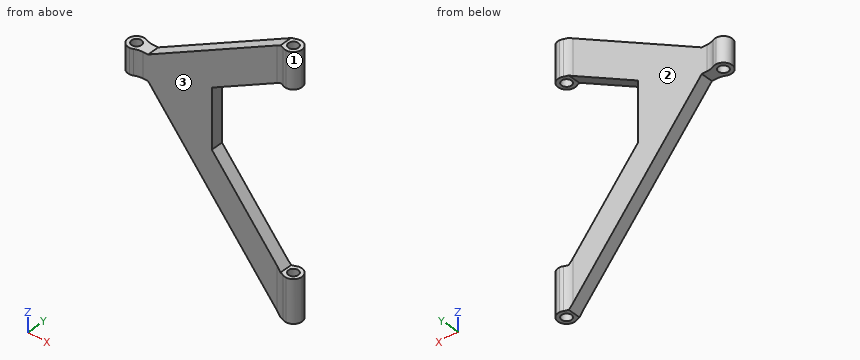
from build123d import *

# Parameters (mm, degrees)
BOSS_EXTRUDE1_DEPTH      = 2.38125
BOSS_EXTRUDE1_DEPTH_BACK = 2.38125
CUT_EXTRUDE1_DEPTH       = 68.891743782
CUT_EXTRUDE1_DEPTH_BACK  = 68.891743782
SKETCH2_R                = 1.375
FILLET2_R                = 2.38125
CUT_EXTRUDE2_DEPTH       = 61.804572212
CUT_EXTRUDE2_DEPTH_BACK  = 61.804572212


with BuildPart() as part:
    # Sketch1 → Boss-Extrude1 (new, two sides: drawn at the far end of the back side and taken through both)
    with BuildSketch(Plane(origin=(0, 0, 0), x_dir=(1, 0, 0), z_dir=(0, 1, 0)).offset(-BOSS_EXTRUDE1_DEPTH_BACK)):
        Polygon((0, 41.898993428), (-37, -2.75), (-44, -2.75), (-44, -9.75), (-37, -9.75), (0, -29.761006572), (4.489108528, -29.761006572), (4.489108528, -19.854089936), (0, -19.854089936), (-19.216520838, -9.461064942), (-19.216520838, 6.902295225), (0, 30.091438809), (4.489108528, 30.091438809), (4.489108528, 41.898993428), align=None)
    extrude(amount=BOSS_EXTRUDE1_DEPTH + BOSS_EXTRUDE1_DEPTH_BACK)

    # Sketch2 → Cut-Extrude1 (cut, two sides: drawn at the far end of the back side and taken through both)
    with BuildSketch(Plane.XY.offset(9.75).offset(-CUT_EXTRUDE1_DEPTH_BACK)):
        with Locations((-41.61875, 0)):
            Circle(SKETCH2_R)
        with Locations((2.107858528, 0)):
            Circle(SKETCH2_R)
    extrude(amount=CUT_EXTRUDE1_DEPTH + CUT_EXTRUDE1_DEPTH_BACK, mode=Mode.SUBTRACT)

    # Fillet2
    fillet2_edges = [part.edges().sort_by_distance(p)[0] for p in [
        (4.489108528, 2.38125, -35.995216119),
        (4.489108528, -2.38125, -35.995216119),
        (4.489108528, -2.38125, 24.807548254),
        (4.489108528, 2.38125, 24.807548254),
        (-44, -2.38125, 6.25),
        (-44, 2.38125, 6.25),
    ]]
    fillet(fillet2_edges, radius=FILLET2_R - 0.0001)  # a hair under: the kernel refuses the full size

    # Sketch3 → Cut-Extrude2 (cut, two sides: drawn at the far end of the back side and taken through both)
    with BuildSketch(Plane.XY.offset(-CUT_EXTRUDE2_DEPTH_BACK)):
        with BuildLine():
            Line((-38.450893086, -1.673565387), (-1.059998386, -1.673565387))
            ThreePointArc((-1.059998386, -1.673565387), (0.043808846, -1.795357088), (1.094509688, -2.154872546))
            ThreePointArc((1.094509688, -2.154872546), (1.588695109, -2.323966632), (2.107858528, -2.38125))
            Line((2.107858528, -2.38125), (2.107858528, -4.833118282))
            Line((2.107858528, -4.833118282), (-41.61875, -4.833118282))
            Line((-41.61875, -4.833118282), (-41.61875, -2.38125))
            ThreePointArc((-41.61875, -2.38125), (-41.099586581, -2.323966632), (-40.60540116, -2.154872546))
            ThreePointArc((-40.60540116, -2.154872546), (-39.554700318, -1.795357088), (-38.450893086, -1.673565387))
        make_face()
        with BuildLine():
            Line((2.107858528, 4.833118282), (2.107858528, 2.38125))
            ThreePointArc((2.107858528, 2.38125), (1.588695109, 2.323966632), (1.094509688, 2.154872546))
            ThreePointArc((1.094509688, 2.154872546), (0.043808846, 1.795357088), (-1.059998386, 1.673565387))
            Line((-1.059998386, 1.673565387), (-38.450893086, 1.673565387))
            ThreePointArc((-38.450893086, 1.673565387), (-39.554700318, 1.795357088), (-40.60540116, 2.154872546))
            ThreePointArc((-40.60540116, 2.154872546), (-41.099586581, 2.323966632), (-41.61875, 2.38125))
            Line((-41.61875, 2.38125), (-41.61875, 4.833118282))
            Line((-41.61875, 4.833118282), (2.107858528, 4.833118282))
        make_face()
    extrude(amount=CUT_EXTRUDE2_DEPTH + CUT_EXTRUDE2_DEPTH_BACK, mode=Mode.SUBTRACT)


solid = part.part
Read the model definition and answer for the solid it produces. Units are mm, in the model's axes. Face numbers are marked on the shaded views. A direction names the side the tool comes from. Round coordinates to 2 decimals unless told otherwise and drop trailing zeros. Write each loop counter-clockwise with the first axis right and the second up, starting at its lowest first coordinate (ties: lowest second). Pieces come first, ordered by that corner, then holes.
Q1. A tool of negligible diameter and unlimited length cuts with its end or side. For the marked faces 1, 2 and 3, from which of +Z, -Z, +X, -X, +Y, -Y can it reach the whole face along a straight path? Write none if from no direction.
Values:
face 1: +Z, -Z, +X, -Y
face 2: +Z, -Z, +Y
face 3: +Z, -Z, -Y
Q2. Find section C-C on z = -22.5. Determine the outline of the cut face in (x, y).
Values:
outline: (-16.08, -1.67) - (-6.29, -1.67) - (-6.29, 1.67) - (-16.08, 1.67) - close
Q3. Find section B-B on x = -24.5. Determine the outline of the cut face in (y, z), and give its area (3 significant figures).
Values:
outline: (-1.67, -12.33) - (1.67, -12.33) - (1.67, 16.51) - (-1.67, 16.51) - close
area: 96.5 mm2
Q4. Flat-ended cylindrical pins translate along their axes: P1, Ø2, axis at x = -41.62, y = 0, coming from the +Z side; P2, Ø2.5, axis at x = -39, y = -0.5, coming from the +Z side; P3, Ø2, axis at x = -30, y = 0, coming from the +Z side; P4, Ø1, axis at x = -25, z = -12, coming from the +Y side. Find the tip coordinate at first contact, or state that the pin passes through.
Values:
P1: passes through
P2: stops at z = 9.75
P3: stops at z = 14.08
P4: stops at y = 1.67
Q5. Find section A-A on x = -9.5. Determine the outline of the cut face in (y, z), and give its area (3 significant figures).
Values:
outline: (-1.67, -30.44) - (1.67, -30.44) - (1.67, -18.63) - (-1.67, -18.63) - close; (-1.67, 14.72) - (1.67, 14.72) - (1.67, 24.62) - (-1.67, 24.62) - close
area: 72.7 mm2
Q6. Straight lines are drawn through the part: line 1 (X direction, y = 0, z = 8.25); line 2 (Y direction, x = -19.5, z = 5.5); line 3 (Z direction, x = -16, y = -0.75). For each, find the intervals that lie inside material, in ascending order.
Values:
line 1: x = -44 to -42.99, -40.24 to -19.22
line 2: y = -1.67 to 1.67
line 3: z = -22.59 to -10.78, 11.2 to 21.11
